from build123d import *

# Parameters (mm, degrees)
SKETCH1_R               = 10.5
BOSS_EXTRUDE1_DEPTH     = 70
SKETCH2_R               = 8.5
CUT_EXTRUDE1_DEPTH      = 0.35
SKETCH3_W               = 21
SKETCH3_H               = 0.25
SKETCH3_W_2             = 0.25
SKETCH3_H_2             = 21
CUT_EXTRUDE_THIN1_DEPTH = 0.25
CUT_EXTRUDE_THIN2_START = 70
SKETCH3_2_W             = 21
SKETCH3_2_H             = 0.25
SKETCH3_2_W_2           = 0.25
SKETCH3_2_H_2           = 21
CUT_EXTRUDE_THIN2_DEPTH = 0.6


with BuildPart() as part:
    # Sketch1 → Boss-Extrude1 (new body)
    with BuildSketch(Plane(origin=(0, 0, 0), x_dir=(1, 0, 0), z_dir=(0, 1, 0))):
        Circle(SKETCH1_R)
    extrude(amount=BOSS_EXTRUDE1_DEPTH)

    # Sketch2 → Cut-Extrude1 (cut)
    with BuildSketch(Plane(origin=(0, 70, 0), x_dir=(1, 0, 0), z_dir=(0, 1, 0))):
        Circle(SKETCH2_R)
    extrude(amount=-CUT_EXTRUDE1_DEPTH, mode=Mode.SUBTRACT)

    # Sketch3 → Cut-Extrude-Thin1 (cut)
    with BuildSketch(Plane(origin=(0, 0, 0), x_dir=(1, 0, 0), z_dir=(0, 1, 0))):
        Rectangle(SKETCH3_W, SKETCH3_H)
        Rectangle(SKETCH3_W_2, SKETCH3_H_2)
    extrude(amount=CUT_EXTRUDE_THIN1_DEPTH, mode=Mode.SUBTRACT)

    # Sketch3<2> → Cut-Extrude-Thin2 (cut)
    with BuildSketch(Plane(origin=(0, 0, 0), x_dir=(1, 0, 0), z_dir=(0, 1, 0)).offset(CUT_EXTRUDE_THIN2_START)):
        with Locations((0, -0.125)):
            Rectangle(SKETCH3_2_W, SKETCH3_2_H)
        with Locations((0.125, 0)):
            Rectangle(SKETCH3_2_W_2, SKETCH3_2_H_2)
    extrude(amount=-CUT_EXTRUDE_THIN2_DEPTH, mode=Mode.SUBTRACT)


solid = part.part
Verification items for the finished model (mm, model axes). A direction names the side the tool comes from. Coordinates: 2 decimals unless noted, no trailing zeros. Loops run counter-clockwise (first coordinate to the right, second up) from the corner with the lowest first, then second, coordinate; pieces in that order, holes last. Notation, with made-up numbers: M 81,55.5 L 138,55.5 A16 ccw 138,71.5 Z; hole C -4.5,42 d1. An arc over 180 degrees is marked long. One line per item, written item: value.
1. Section check C-C on y = 47.5. Record the cut outline in (x, z), plus the area to 3 significant figures.
Answers follow:
outline: C 0,0 d21
area: 346 mm^2
2. Mould release check, pull along X, two halves, no side actions. Record for faces 1 (the cylindrical face through (-5.94, 69.83, -6.08)), 2 (the cylindrical face through (10, 34.5, -3.2)), 3 (the flat face through (6.1, 70, 6.5)): pulls with the +X half, pulls with the -X half, needs draft (parallel to the pull), parting line crosses it, or undercut.
Answers follow:
face 1: undercut
face 2: parting line crosses it
face 3: needs draft
3. Gauge pin test, flat ends, axial feed: P1, Ø2, axis at y = 55.5, z = -7, coming from the +X side; P2, Ø6, axis at y = 57.5, z = -7.5, coming from the -X side; P3, Ø2, axis at x = -7, y = 19, coming from the +Z side. Record the tip position at first contact, or that the pin passes through.
Answers follow:
P1: x = 8.62
P2: x = -9.49
P3: z = 8.62
4. Material ranges on line 1 along Y through (x, z) = (0.5, 7.5); line 2 along X through (y, z) = (48.5, 8.25); line 3 along Z through (x, y) = (0.75, 54), recorded low to high. Write a range as from..to.
Answers follow:
line 1: 0..69.65
line 2: -6.5..6.5
line 3: -10.47..10.47
5. Section check B-B on x = -7.5. Record the cut outline in (y, z) (3 decimals).
Answers follow:
outline: M 0,-7.348 L 70,-7.348 L 70,-4 L 69.65,-4 L 69.65,0 L 69.4,0 L 69.4,0.25 L 69.65,0.25 L 69.65,4 L 70,4 L 70,7.348 L 0,7.348 L 0,0.125 L 0.25,0.125 L 0.25,-0.125 L 0,-0.125 Z
6. Set-up check for faces 4 (the cylindrical face through (5.95, 69.83, 6.07)), 5 (the flat face through (-6.1, 70, 6.5)): record each of +Z, -Z, +X, -X, +Y, -Y from which the full face is reachable in a straight line by a thin tool's end or side.
Answers follow:
face 4: +Y
face 5: +Z, -Z, +X, -X, +Y
7. Section check A-A on z = -3. Record the cut outline in (x, y) (3 decimals).
Answers follow:
outline: M -10.062,0 L -0.125,0 L -0.125,0.25 L 0.125,0.25 L 0.125,0 L 10.062,0 L 10.062,70 L 7.953,70 L 7.953,69.65 L 0.25,69.65 L 0.25,69.4 L 0,69.4 L 0,69.65 L -7.953,69.65 L -7.953,70 L -10.062,70 Z
